Build history of the part. All positions in model axes, mm. Round coordinates to 2 decimals unless told otherwise and drop trailing zeros. Write each loop counter-clockwise with the first axis right and the second up, starting at its lowest first coordinate (ties: lowest second). Pieces come first, ordered by that corner, then holes. Notation, with made-up numbers: (30, 3) - (72, 3) arc R22 cw to (72, 9) - close; hole circle Ø7 at (77, 48.5). An arc over 180 degrees is marked (long way). Write each question's results on one line, items separated by ' | '.
from build123d import *

# Parameters (mm, degrees)
SKETCH1_R           = 49.53
BOSS_EXTRUDE1_DEPTH = 3.175
SKETCH2_R           = 3.175
CUT_EXTRUDE1_DEPTH  = 263.398
SKETCH3_R           = 3.175
CUT_EXTRUDE2_DEPTH  = 25.4
SKETCH4_R           = 1.5875
SKETCH4_R_2         = 1.25
CUT_EXTRUDE3_DEPTH  = 50.8


with BuildPart() as part:
    # Sketch1 → Boss-Extrude1 (new body)
    with BuildSketch(Plane(origin=(0, 0, 0), x_dir=(1, 0, 0), z_dir=(0, 1, 0))):
        Circle(SKETCH1_R)
    extrude(amount=BOSS_EXTRUDE1_DEPTH)

    # Sketch2 → Cut-Extrude1 (cut)
    with BuildSketch(Plane(origin=(-55.039702575, 234.95, -116.088398355), x_dir=(-1, 0, 0), z_dir=(0, 1, 0))):
        with Locations((-93.139702575, 116.088398355)):
            Circle(SKETCH2_R)
        with Locations((-16.939702575, 116.088398355)):
            Circle(SKETCH2_R)
    extrude(amount=-CUT_EXTRUDE1_DEPTH, mode=Mode.SUBTRACT)

    # Sketch3 → Cut-Extrude2 (cut)
    with BuildSketch(Plane(origin=(-28.264398128, 0, -82.371298873), x_dir=(1, 0, 0), z_dir=(0, -1, 0))):
        with Locations((28.264398128, 98.246298873)):
            Circle(SKETCH3_R)
        with Locations((28.264398128, 66.496298873)):
            Circle(SKETCH3_R)
    extrude(amount=-CUT_EXTRUDE2_DEPTH, mode=Mode.SUBTRACT)

    # Sketch4 → Cut-Extrude3 (cut)
    with BuildSketch(Plane(origin=(-28.264398128, 0, -82.371298873), x_dir=(-1, 0, 0), z_dir=(0, -1, 0))):
        with Locations((-3.404148128, -108.914298873)):
            Circle(SKETCH4_R)
        with Locations((-12.802148128, -108.914298873)):
            Circle(SKETCH4_R)
        with Locations((-43.726648128, -108.914298873)):
            Circle(SKETCH4_R)
        with Locations((-53.124648128, -108.914298873)):
            Circle(SKETCH4_R)
        with Locations((-8.103148128, -97.230298873)):
            Circle(SKETCH4_R_2)
        with Locations((-48.425648128, -97.230298873)):
            Circle(SKETCH4_R_2)
    extrude(amount=-CUT_EXTRUDE3_DEPTH, mode=Mode.SUBTRACT)


solid = part.part
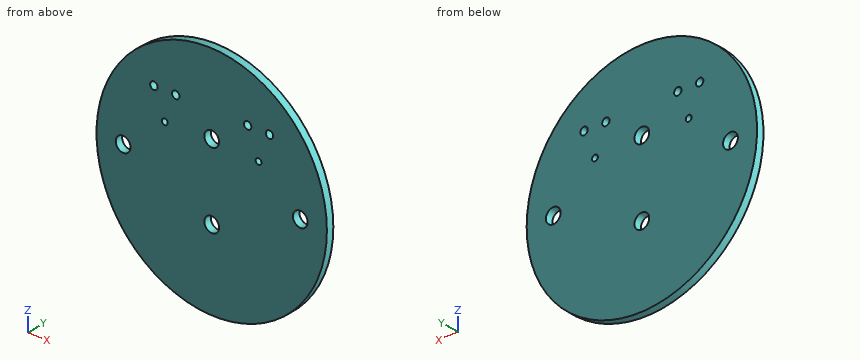
(1) Flat gauge pins, fed straight in: pin 1 Ø4 at (x, z) = (38.1, 0) entering from +Y; pin 2 Ø1 at (x, y) = (27, 1) entering from +Z; pin 3 Ø1.5 at (x, y) = (-9.5, 1.5) entering from -Z. Where does each tip first touch, or does it go through?
Worked answers:
pin 1: passes through | pin 2: stops at z = 41.84 | pin 3: stops at z = -48.75
(2) Slice it at B-B, the plane x = 0. Write the cut outline in (y, z) (3 decimals).
Worked answers:
outline: (0, -49.53) - (3.175, -49.53) - (3.175, -19.05) - (0, -19.05) - close; (0, -12.7) - (3.175, -12.7) - (3.175, 12.7) - (0, 12.7) - close; (0, 19.05) - (3.175, 19.05) - (3.175, 49.53) - (0, 49.53) - close
(3) Slice it at C-C, the plane y = 0.85. State how many separate pieces and enclosed holes the cut face has, and give its area (3 significant figures).
Worked answers:
separate pieces: 1 | enclosed holes: 10 | area: 7,540 mm2
(4) Slice it at A-A, the plane z = 0. Write the cut outline in (x, y) (3 decimals), and give its area (3 significant figures).
Worked answers:
outline: (-49.53, 0) - (-41.275, 0) - (-41.275, 3.175) - (-49.53, 3.175) - close; (-34.925, 0) - (34.925, 0) - (34.925, 3.175) - (-34.925, 3.175) - close; (41.275, 0) - (49.53, 0) - (49.53, 3.175) - (41.275, 3.175) - close | area: 274 mm2
(5) Slice it at D-D, the plane x = 38.1. Write the cut outline in (y, z) (3 decimals).
Worked answers:
outline: (0, -31.648) - (3.175, -31.648) - (3.175, -3.175) - (0, -3.175) - close; (0, 3.175) - (3.175, 3.175) - (3.175, 31.648) - (0, 31.648) - close
(6) Drill centre lines: probe 1 along Z at (x, y) = (0, 1.7); probe 2 along X at (y, z) = (1.95, 15); probe 3 along Z at (x, y) = (-36.5, 2.45). Where is each one in solid material? Low to high. Write a range as [from, to].
Worked answers:
probe 1: z = [-49.53, -19.05], [-12.7, 12.7], [19.05, 49.53] | probe 2: x = [-47.2, -21.4], [-18.92, -3.05], [3.05, 18.92], [21.4, 47.2] | probe 3: z = [-33.48, -2.74], [2.74, 33.48]
